The listing builds one solid part. Answer for the finished solid, in the listing's coordinates (mm). A direction names the side the tool comes from. Coordinates: 2 decimals unless noted, no trailing zeros. Loops run counter-clockwise (first coordinate to the right, second up) from the corner with the lowest first, then second, coordinate; pieces in that order, holes last. Notation, with made-up numbers: M -19.5,-14.5 L -4.5,-14.5 A8 ccw -4.5,-7.5 Z; hole C 85,21.25 d2. An arc over 180 degrees is marked long. Return JSON: item names as keys, results as strings. Group by question number.
1. The mould has two halves that part along Z. Classify faces 3 (the face through (-38.78, -25, 9)), 4 (the face through (-32, -25, 49.753)), 5 (the face through (-13.897, -24.65, 28.532)): pulls with the +Z half, pulls with the -Z half, needs draft (parallel to the pull), parting line crosses it, or undercut.
2. Straight lines are drawn through the part: L1, parallel to X at y = -42, z = 48; L2, parallel to Z at x = -33, y = -45.5; L3, parallel to Z at x = -31, y = -43. For each, find the intervals that lie inside material, in ascending order. Write a range as from..to.
3. Section A-A (z = 49) is taken. Write down the section's boundary in (x, y).
4. Given P1, Ø6.5, axis at y = -26.5, z = 6.5, coming from the +X side; P2, Ø9, axis at x = -5, y = -13, coming from the +Z side; P3, Ø3, axis at y = -31.5, z = 51, coming from the +X side, each flat-ended and moving along its own axis, determine where each tip first touches the part or whether it passes through.
5. Section C-C (x = -6) is taken. Write down the section's boundary in (y, z) (3 decimals).
6. Which of the six approach directions +Z, -Z, +X, -X, +Y, -Y give full straight-line access (tool end or side, diameter ignored) to faces 1 (the face through (-18, -50, 27)), 2 (the face through (-33.83, -24.65, 21.47))?
7. Section B-B (x = -32.5) is taken. Write down the section's boundary in (y, z), then the cut area to 3 significant figures.
```python
from build123d import *

# Parameters (mm, degrees)
F1_DEPTH = 50


with BuildPart() as f1:
    # F0 (on Front) → F1 (new body)
    with BuildSketch(Plane.XZ):
        Polygon((-39.080582, 53.752999), (-39.080582, 29.963545), (-36.328474, 25.460097), (-38.779549, 20.467168), (-38.779549, -3.381329), (3.029354, -3.381329), (2.930473, 19.121045), (-0.091638, 23.40237), (-11.598663, 23.40237), (-16.2607, 33.807004), (-24.053911, 41.383733), (-25.210454, 43.429926), (-25.210454, 53.752999), align=None)
        Polygon((-1.063952, 17.843597), (-0.988262, 0.618671), (-34.779549, 0.618671), (-34.779549, 13.328114), (-34.026969, 16.037403), (-35.833161, 17.392047), (-31.769227, 25.67043), (-35.080582, 31.089008), (-35.080582, 49.752999), (-29.210454, 49.752999), (-29.210454, 42.377714), (-27.253745, 38.915843), (-21.835167, 33.647783), (-19.42691, 33.647783), (-20.330006, 29.734364), (-19.727943, 28.229203), (-21.233102, 26.272494), (-19.727943, 25.114681), (-17.470201, 26.724044), (-14.737966, 22.891048), (-14.008333, 20.101337), (-12.20214, 19.348757), (-11.148528, 17.241532), (-4.224789, 18.295145), (-2.870144, 20.40237), align=None, mode=Mode.SUBTRACT)
    extrude(amount=F1_DEPTH)


solid = f1.part
```
Worked out:
{
 "1": {"face 3": "needs draft", "face 4": "undercut", "face 5": "pulls with the +Z half"},
 "2": {"L1": "-39.08..-35.08, -29.21..-25.21", "L2": "-3.38..0.62, 23.16..27.68, 49.75..53.75", "L3": "-3.38..0.62, 49.75..53.75"},
 "3": {"outline": "M -39.08,-50 L -35.08,-50 L -35.08,0 L -39.08,0 Z; M -29.21,-50 L -25.21,-50 L -25.21,0 L -29.21,0 Z"},
 "4": {"P1": "x = 3", "P2": "z = 23.4", "P3": "x = -25.21"},
 "5": {"outline": "M -50,-3.381 L 0,-3.381 L 0,0.619 L -50,0.619 Z; M -50,18.025 L 0,18.025 L 0,23.402 L -50,23.402 Z"},
 "6": {"face 1": "+Z, -Z, +X, -X, -Y", "face 2": "+Y, -Y"},
 "7": {"outline": "M -50,-3.38 L 0,-3.38 L 0,0.62 L -50,0.62 Z; M -50,24.18 L 0,24.18 L 0,26.87 L -50,26.87 Z; M -50,49.75 L 0,49.75 L 0,53.75 L -50,53.75 Z", "area": "534 mm^2"}
}
